Geometry: final body of the model. Coordinates: model frame, mm. Round coordinates to 2 decimals unless told otherwise and drop trailing zeros. Order: outer loops, then holes, each group sorted by start corner. A loop starts at its lowest first (then second) coordinate and runs counter-clockwise, first axis right, second up. Notation, with made-up numbers: M 72.5,29 L 93.5,29 A11 ccw 93.5,38 Z; hole C -13.5,35.5 d10. An arc over 180 degrees is marked long. Return JSON: item names as keys, results as strings. Group by question number.
Q1. Cut plane A-A on y = 0. Count the separate pieces of the cut face and the enclosed holes in it, and give its area (3 significant figures).
Q2. Ray query, probe 1 along Z at (x, y) = (-6.75, -0.5); probe 2 along Y at (x, z) = (-0.75, -30); probe 3 along Z at (x, y) = (8, 2). Return the intervals inside material, ascending.
Q3. Contact query for flat-ended pins moving along their axis: pin 1 (9 mm diameter, centred on y = 0, z = -30, fed in from +X); pin 2 (3 mm diameter, centred on x = -5, z = -516, fed in from +Y); pin 3 (3 mm diameter, centred on x = -6.5, z = -726.5, fed in from -Y). Output: stop coordinate, or through.
Q4. Cut plane B-B on z = -360. Output: boundary loops of the cut face in (x, y), and give its area (3 significant figures).
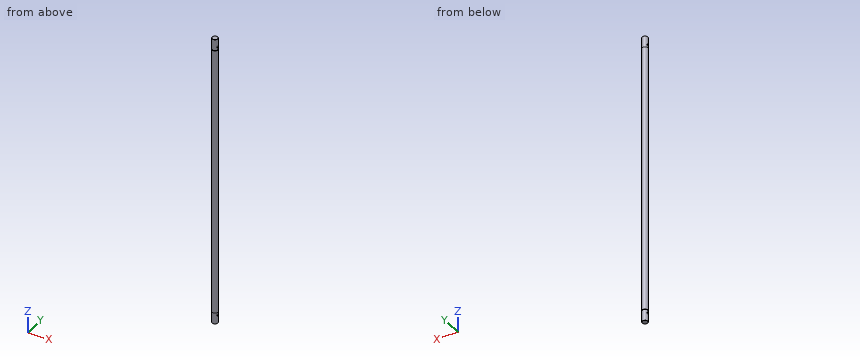
```python
from build123d import *

# Parameters (mm, degrees)
SKETCH_2_R          = 4
CUT_EXTRUDE_1_DEPTH = 1035.271724452
SKETCH_3_R          = 4
CUT_EXTRUDE_2_DEPTH = 1035.271724452
FILLET_1_R          = 0.2
CHAMFER_1_SIZE      = 0.5


with BuildPart() as part:
    # Эскиз1 → Повернуть1 (revolve)
    with BuildSketch(Plane(origin=(0, 0, 0), x_dir=(0, 0, -1), z_dir=(1, 0, 0)), mode=Mode.PRIVATE) as revolve_1_sk:
        Polygon((0, 0), (0, 10), (40, 10), (40, 11), (994, 11), (994, 10), (1034, 10), (1034, 0), align=None)
    revolve(revolve_1_sk.sketch.rotate(Axis((0, 0, 0), (0, 0, -1)), 90), axis=Axis((0, 0, 0), (0, 0, -1)))

    # Эскиз2 → Вырез-Вытянуть1 (cut, through all)
    with BuildSketch(Plane.ZY.offset(10)):
        with Locations((-30, 0)):
            Circle(SKETCH_2_R)
    extrude(amount=-CUT_EXTRUDE_1_DEPTH, mode=Mode.SUBTRACT)

    # Эскиз3 → Вырез-Вытянуть2 (cut, through all)
    with BuildSketch(Plane.ZY.offset(10)):
        with Locations((-1004, 0)):
            Circle(SKETCH_3_R)
    extrude(amount=-CUT_EXTRUDE_2_DEPTH, mode=Mode.SUBTRACT)

    # Скругление1
    fillet_1_edges = [part.edges().sort_by_distance(p)[0] for p in [
        (-10, 0, -994),
        (-10, 0, -40),
    ]]
    fillet(fillet_1_edges, radius=FILLET_1_R)

    # Фаска1
    chamfer_1_edges = [part.edges().sort_by_distance(p)[0] for p in [
        (-10, 0, -1034),
        (-11, 0, -994),
        (-11, 0, -40),
        (-10, 0, 0),
    ]]
    chamfer(chamfer_1_edges, length=CHAMFER_1_SIZE)


solid = part.part
```
Result sheet:
{
 "1": {"separate pieces": "3", "enclosed holes": "0", "area": "22,300 mm²"},
 "2": {"probe 1": "z = -1034 to -1007.97, -1000.03 to -33.97, -26.03 to 0", "probe 2": "y = -9.97 to -4, 4 to 9.97", "probe 3": "z = -1034 to -1007.46, -1000.54 to -33.46, -26.54 to 0"},
 "3": {"pin 1": "stops at x = 10", "pin 2": "stops at y = 10.43", "pin 3": "stops at y = -9.8"},
 "4": {"outline": "C 0,0 d22", "area": "380 mm²"}
}
